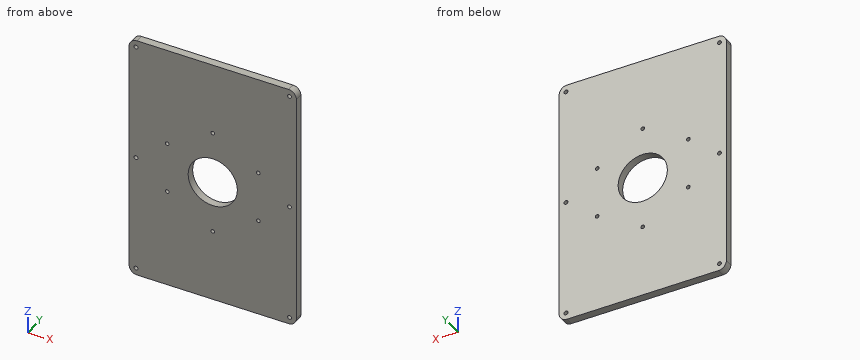
from build123d import *

# Parameters (mm, degrees)
SKETCH1_W             = 170
SKETCH1_H             = 250
BOSS_EXTRUDE1_DEPTH   = 8
SKETCH3_R             = 2
CUT_EXTRUDE2_DEPTH    = 8
FILLET1_R             = 8
CROQUIS1_R            = 25
CROQUIS1_R_2          = 1.866016506
CORTAR_EXTRUIR3_DEPTH = 10


with BuildPart() as part:
    # Sketch1 → Boss-Extrude1 (new body)
    with BuildSketch(Plane(origin=(0, 0, 0), x_dir=(1, 0, 0), z_dir=(0, 1, 0))):
        Rectangle(SKETCH1_W, SKETCH1_H)
    extrude(amount=BOSS_EXTRUDE1_DEPTH)

    # Sketch3 → Cut-Extrude2 (cut)
    with BuildSketch(Plane(origin=(0, 8, 0), x_dir=(1, 0, 0), z_dir=(0, 1, 0))):
        with Locations(Location((-78, 118, 0), (0, 0, 270))):
            Circle(SKETCH3_R)
        with Locations(Location((78, 118, 0), (0, 0, 90))):
            Circle(SKETCH3_R)
        with Locations(Location((78, -118, 0), (0, 0, 270))):
            Circle(SKETCH3_R)
        with Locations(Location((-78, -118, 0), (0, 0, 90))):
            Circle(SKETCH3_R)
        with Locations(Location((-78, 0, 0), (0, 0, 270))):
            Circle(SKETCH3_R)
        with Locations(Location((78, 0, 0), (0, 0, 90))):
            Circle(SKETCH3_R)
    extrude(amount=-CUT_EXTRUDE2_DEPTH, mode=Mode.SUBTRACT)

    # Fillet1
    fillet1_edges = [part.edges().sort_by_distance(p)[0] for p in [
        (85, 4, 125),
        (-85, 4, 125),
        (-85, 4, -125),
        (85, 4, -125),
    ]]
    fillet(fillet1_edges, radius=FILLET1_R)

    # Croquis1 → Cortar-Extruir3 (cut)
    with BuildSketch(Plane(origin=(0, 8, 0), x_dir=(1, 0, 0), z_dir=(0, 1, 0))):
        with Locations(Location((0, 0, 0), (0, 0, 270))):
            Circle(CROQUIS1_R)
        with Locations(Location((0, 52.412836982, 0), (0, 0, 270))):
            Circle(CROQUIS1_R_2)
        with Locations(Location((-46.34372748, 25.540560465, 0), (0, 0, 270))):
            Circle(CROQUIS1_R_2)
        with Locations(Location((0, -52.412836982, 0), (0, 0, 270))):
            Circle(CROQUIS1_R_2)
        with Locations(Location((-46.34372748, -25.540560465, 0), (0, 0, 270))):
            Circle(CROQUIS1_R_2)
        with Locations(Location((46.34372748, 25.540560465, 0), (0, 0, 270))):
            Circle(CROQUIS1_R_2)
        with Locations(Location((46.34372748, -25.540560465, 0), (0, 0, 270))):
            Circle(CROQUIS1_R_2)
    extrude(amount=-CORTAR_EXTRUIR3_DEPTH, mode=Mode.SUBTRACT)


solid = part.part
Check sheet for the modelled part. Datum: model origin and axes. Units: mm. Round coordinates to 2 decimals unless told otherwise and drop trailing zeros. Order: outer loops, then holes, each group sorted by start corner. A loop starts at its lowest first (then second) coordinate and runs counter-clockwise, first axis right, second up.
Q1. Cross-section at C-C, the plane x = -19. Enter the section's corners in (y, z), plus the area to 3 significant figures.
Filled sheet:
outline: (0, -125) - (8, -125) - (8, -16.25) - (0, -16.25) - close; (0, 16.25) - (8, 16.25) - (8, 125) - (0, 125) - close
area: 1,740 mm2
Q2. Cross-section at B-B, the plane y = 6.5. Give the number of separate pieces and of enclosed holes in the cut face, plus the area to 3 significant figures.
Filled sheet:
separate pieces: 1
enclosed holes: 13
area: 40,300 mm2
Q3. Depth check by flat-ended pin: P1, Ø3, axis at x = -30, z = 5, coming from the -Y side. Enter the tip coordinate at first touch or a pass-through.
Filled sheet:
P1: stops at y = 0
Q4. Scan lines: L1, parallel to X at y = 2.5, z = 0; L2, parallel to Z at x = -10, y = 1.5; L3, parallel to Z at x = -3, y = 7. Record each from-to range of solid material in increasing order.
Filled sheet:
L1: x = -85 to -80, -76 to -25, 25 to 76, 80 to 85
L2: z = -125 to -22.91, 22.91 to 125
L3: z = -125 to -24.82, 24.82 to 125
Q5. Cross-section at A-A, the plane x = 17. Enter the section's corners in (y, z).
Filled sheet:
outline: (0, -125) - (8, -125) - (8, -18.33) - (0, -18.33) - close; (0, 18.33) - (8, 18.33) - (8, 125) - (0, 125) - close
